Input: part model. Units: mm. Frame: model coordinates. A direction names the side the tool comes from. Coordinates: 2 decimals unless noted, no trailing zeros. Write each loop counter-clockwise with the first axis right and the second up, starting at its lowest first coordinate (ties: lowest second). Pieces come first, ordered by that corner, then holes. Notation, with made-up numbers: (2, -21.5) -> (26, -21.5) arc R27 cw to (26, 8.5) -> close; hole circle Ø10 at (60.25, -20). An arc over 180 degrees is marked (long way). Use one line per item in the form item = value. Start each with the question number.
(1) First-contact query: pin 1 (8 mm diameter, centred on x = 145.5, y = 19, fed in from -Z); pin 2 (1.6 mm diameter, centred on x = 65, y = 20, fed in from -Z); pin 3 (5 mm diameter, centred on y = 39, z = 98, fed in from +X); pin 4 (5 mm diameter, centred on y = 10.5, z = 191, fed in from +X). Flat tips, straight axial feed; report the tip coordinate or a pass-through.
(2) Cut plane D-D on x = -225.5. Return the cut outline in (y, z), plus the area to 3 significant figures.
(3) Ray query, line 1 along X through (y, z) = (32, 0); line 2 along Z through (x, y) = (0, 23); line 3 along Z through (x, y) = (0, 14). Return the intervals inside material, ascending.
(4) Pull-direction query (X, two-part tool) for faces 1 (the face through (482.905, 35, 0)), 2 (the face through (-62.446, 34.51, -2.608)), 3 (the face through (0, 35, -482.905)); classes: released by +X, released by -X, zero draft, split by the parting line, or undercut.
(5) Cut plane B-B on y = 35. Return the cut outline in (x, z), plus the area to 3 significant figures.
(6) Set-up query: faces 4 (the face through (2.6, 54.83, -278.65)), 5 (the face through (-278.65, 54.83, -2.6)), 6 (the face through (278.65, 54.83, 2.6)), 7 (the face through (-2.6, 54.83, 278.65)). Return all of +Z, -Z, +X, -X, +Y, -Y with unobstructed straight access to the full face (end or side cutting, diameter ignored); none if empty.
(7) Cut plane A-A on x = 0. Return the cut outline in (y, z), plus the area to 3 significant figures.
(8) Cut plane C-C on z = -300.5. Return the cut outline in (x, y), plus the area to 3 significant figures.
```python
from build123d import *

# Parameters (mm, degrees)
IZIM1_R                     = 82.5
IZIM1_R_2                   = 62.5
Y_KSEKLIK_EKSTR_ZYON1_DEPTH = 70
IZIM2_R                     = 20
Y_KSEKLIK_EKSTR_ZYON2_DEPTH = 405
DAIRESEL_KAPLAMA1_COUNT     = 4
IZIM4_W                     = 15
IZIM4_H                     = 20
KES_EKSTR_ZYON1_DEPTH       = 71.0000001


with BuildPart() as part:
    # Çizim1 → Yükseklik-Ekstrüzyon1 (new body)
    with BuildSketch(Plane(origin=(0, 0, 0), x_dir=(1, 0, 0), z_dir=(0, 1, 0))):
        Circle(IZIM1_R)
        Circle(IZIM1_R_2, mode=Mode.SUBTRACT)
    extrude(amount=Y_KSEKLIK_EKSTR_ZYON1_DEPTH)

    # Çizim2 → Yükseklik-Ekstrüzyon2 (add)
    with BuildSketch(Plane(origin=(77.904802992, 0, 0), x_dir=(0, 0, -1), z_dir=(1, 0, 0))):
        with Locations((0, 35)):
            Circle(IZIM2_R)
    y_kseklik_ekstr_zyon2 = extrude(amount=Y_KSEKLIK_EKSTR_ZYON2_DEPTH)

    # Dairesel Kaplama1: Yükseklik-Ekstrüzyon2 ×4 about axis
    dairesel_kaplama1_axis = Axis((0, 0, 0), (0, 1, 0))
    for i in range(1, DAIRESEL_KAPLAMA1_COUNT):
        add(y_kseklik_ekstr_zyon2.rotate(dairesel_kaplama1_axis, i * 360 / DAIRESEL_KAPLAMA1_COUNT))

    # Çizim4 → Kes-Ekstrüzyon1 (cut, through all)
    with BuildSketch(Plane(origin=(0, 70, 0), x_dir=(1, 0, 0), z_dir=(0, 1, 0))):
        with Locations((59.5, 0)):
            Rectangle(IZIM4_W, IZIM4_H)
    extrude(amount=-KES_EKSTR_ZYON1_DEPTH, mode=Mode.SUBTRACT)


solid = part.part
```
Values:
q1.pin_1 = -16
q1.pin_2 = -51.81
q1.pin_3 = 19.94
q1.pin_4 = through
q2.outline = circle Ø40 at (35, 0)
q2.area = 1,260 mm2
q3.line_1 = -482.9 to -62.5, 67 to 482.9
q3.line_2 = -482.9 to -62.5, 62.5 to 482.9
q3.line_3 = -82.5 to -62.5, 62.5 to 82.5
q4.face_1 = released by +X
q4.face_2 = undercut
q4.face_3 = zero draft
q5.outline = (-482.9, -20) -> (-80.04, -20) arc R82.5 ccw to (-20, -80.04) -> (-20, -482.9) -> (20, -482.9) -> (20, -80.04) arc R82.5 ccw to (80.04, -20) -> (482.9, -20) -> (482.9, 20) -> (80.04, 20) arc R82.5 ccw to (20, 80.04) -> (20, 482.9) -> (-20, 482.9) -> (-20, 80.04) arc R82.5 ccw to (-80.04, 20) -> (-482.9, 20) -> close; hole (61.69, -10) -> (67, -10) -> (67, 10) -> (61.69, 10) arc R62.5 ccw (long way) to start
q5.area = 73,200 mm2
q6.face_4 = -Z
q6.face_5 = -X
q6.face_6 = +X
q6.face_7 = +Z
q7.outline = (0, -82.5) -> (15, -82.5) -> (15, -482.9) -> (55, -482.9) -> (55, -82.5) -> (70, -82.5) -> (70, -62.5) -> (0, -62.5) -> close; (0, 62.5) -> (70, 62.5) -> (70, 82.5) -> (55, 82.5) -> (55, 482.9) -> (15, 482.9) -> (15, 82.5) -> (0, 82.5) -> close
q7.area = 34,800 mm2
q8.outline = circle Ø40 at (0, 35)
q8.area = 1,260 mm2
